```python
from build123d import *

# Parameters (mm, degrees)
EXTRUDE_1_DEPTH     = 5
SKETCH_1_12_R       = 1.5
CUT_EXTRUDE_1_DEPTH = 116.382644488
CUT_EXTRUDE_START   = 5
SKETCH_1_13_R       = 2.25
CUT_EXTRUDE_3_DEPTH = 3


with BuildPart() as part:
    # 草图1 → 凸台-拉伸1 (new body)
    with BuildSketch(Plane(origin=(0, 0, 0), x_dir=(1, 0, 0), z_dir=(0, 1, 0))):
        Polygon((-28.642135833, 0), (0, 0), (0, 91.231745931), (-12.313708499, 91.231745931), (-12.313708499, 98.231745931), (0, 98.231745931), (0, 111.65922579), (-28.642135833, 111.65922579), align=None)
    extrude(amount=EXTRUDE_1_DEPTH)

    # 草图1<12> → 切除-拉伸1 (cut, through all)
    with BuildSketch(Plane(origin=(0, 0, 0), x_dir=(1, 0, 0), z_dir=(0, 1, 0))):
        with Locations(Location((-20.313708499, 83.231745931, 0), (0, 0, 270))):
            Circle(SKETCH_1_12_R)
        with Locations(Location((-20.313708499, 16.763708499, 0), (0, 0, 270))):
            Circle(SKETCH_1_12_R)
        with Locations(Location((-9, 5.45, 0), (0, 0, 270))):
            Circle(SKETCH_1_12_R)
    extrude(amount=CUT_EXTRUDE_1_DEPTH, mode=Mode.SUBTRACT)

    # 草图1<13> → 切除-拉伸3 (cut)
    with BuildSketch(Plane(origin=(0, 0, 0), x_dir=(1, 0, 0), z_dir=(0, 1, 0)).offset(CUT_EXTRUDE_START)):
        with Locations(Location((-20.313708499, 83.231745931, 0), (0, 0, 270))):
            Circle(SKETCH_1_13_R)
        with Locations(Location((-9, 5.45, 0), (0, 0, 270))):
            Circle(SKETCH_1_13_R)
        with Locations(Location((-20.313708499, 16.763708499, 0), (0, 0, 270))):
            Circle(SKETCH_1_13_R)
    extrude(amount=-CUT_EXTRUDE_3_DEPTH, mode=Mode.SUBTRACT)


solid = part.part
```
Build history of the part. All positions in model axes, mm. A direction names the side the tool comes from. Coordinates: 2 decimals unless noted, no trailing zeros. Order: outer loops, then holes, each group sorted by start corner. A loop starts at its lowest first (then second) coordinate and runs counter-clockwise, first axis right, second up.
Item 1: Saw through at C-C on x = -9. List the corners of the cut face in (y, z), then the cut area to 3 significant figures.
Filled in:
outline: (0, -111.66) - (5, -111.66) - (5, -98.23) - (0, -98.23) - close; (0, -91.23) - (5, -91.23) - (5, -7.7) - (2, -7.7) - (2, -6.95) - (0, -6.95) - close; (0, -3.95) - (2, -3.95) - (2, -3.2) - (5, -3.2) - (5, 0) - (0, 0) - close
area: 504 mm2
Item 2: Saw through at B-B on z = -5.45. List the corners of the cut face in (x, y), then the cut area to 3 significant figures.
Filled in:
outline: (-28.64, 0) - (-10.5, 0) - (-10.5, 2) - (-11.25, 2) - (-11.25, 5) - (-28.64, 5) - close; (-7.5, 0) - (0, 0) - (0, 5) - (-6.75, 5) - (-6.75, 2) - (-7.5, 2) - close
area: 124 mm2
Item 3: Mould opens along Z. For faces 4 (the flat face through (-6, 2, -91.232)), 5 (the flat face through (-15, 5, -57)), 6 (the flat face through (-15, 2, 0)), 7 (the flat face through (-6, 2, -98.232)) say: released by +Z, released by -Z, zero draft, split by the parting line, or undercut.
Filled in:
face 4: undercut
face 5: zero draft
face 6: released by +Z
face 7: undercut
Item 4: Drop flat-ended pins along their axis: pin 1 Ø4 at (x, z) = (-9, -5.45) entering from +Y; pin 2 Ø2.5 at (y, z) = (2, -94.5) entering from +X. Give the stop position or say it passes through.
Filled in:
pin 1: stops at y = 2
pin 2: stops at x = -12.31
Item 5: Drill centre lines: L1, parallel to Z at x = -8.75, y = 1; L2, parallel to X at y = 1.15, z = -5.45; L3, parallel to Z at x = -20.5, y = 1.55. Where is each one in solid material? Low to high.
Filled in:
L1: z = -111.66 to -98.23, -91.23 to -6.93, -3.97 to 0
L2: x = -28.64 to -10.5, -7.5 to 0
L3: z = -111.66 to -84.72, -81.74 to -18.25, -15.28 to 0
Item 6: Tool access for faces 1 (the flat face through (-15, 0, -57)), 2 (the flat face through (-22, 2, -83)), 3 (the flat face through (-12.314, 2, -95)): list every direction of +Z, -Z, +X, -X, +Y, -Y with a clear straight run to the whole face (end or side of a thin tool).
Filled in:
face 1: +Z, -Z, +X, -X, -Y
face 2: +Y
face 3: +X, +Y, -Y
Item 7: Saw through at A-A on x = -3.5. List the corners of the cut face in (y, z).
Filled in:
outline: (0, -111.66) - (5, -111.66) - (5, -98.23) - (0, -98.23) - close; (0, -91.23) - (5, -91.23) - (5, 0) - (0, 0) - close
Item 8: Saw through at D-D on y = 2.8. List the corners of the cut face in (x, z).
Filled in:
outline: (-28.64, -111.66) - (0, -111.66) - (0, -98.23) - (-12.31, -98.23) - (-12.31, -91.23) - (0, -91.23) - (0, 0) - (-28.64, 0) - close; hole circle Ø4.5 at (-20.31, -83.23); hole circle Ø4.5 at (-20.31, -16.76); hole circle Ø4.5 at (-9, -5.45)
